```python
from build123d import *

# Parameters (mm, degrees)
ESQUISSE1_R                  = 250
BOSS_EXTRU_1_DEPTH           = 5
D_GAGEMENT_M101_D            = 12
D_GAGEMENT_M101_CSINK_D      = 12.05
D_GAGEMENT_M101_CSINK_ANGLE  = 90
ESQUISSE6_R                  = 1.25
ENL_V_MAT_EXTRU_1_DEPTH      = 11
R_P_TITION_CIRCULAIRE1_COUNT = 3


with BuildPart() as part:
    # Esquisse1 → Boss.-Extru.1 (new body, symmetric)
    with BuildSketch(Plane(origin=(0, 0, 0), x_dir=(1, 0, 0), z_dir=(0, 1, 0))):
        Circle(ESQUISSE1_R)
    extrude(amount=BOSS_EXTRU_1_DEPTH, both=True)

    # Dégagement M101 (through all)
    with Locations(Plane(origin=(0, 5, 0), x_dir=(1, 0, 0), z_dir=(0, 1, 0))):
        with Locations((0, 0)):
            CounterSinkHole(D_GAGEMENT_M101_D / 2, D_GAGEMENT_M101_CSINK_D / 2, counter_sink_angle=D_GAGEMENT_M101_CSINK_ANGLE)

    # Esquisse6 → Enlèv. mat.-Extru.1 (cut, through all)
    with BuildSketch(Plane(origin=(0, 5, 0), x_dir=(1, 0, 0), z_dir=(0, 1, 0))):
        with Locations((200, 8)):
            Circle(ESQUISSE6_R)
        with Locations((200, -8)):
            Circle(ESQUISSE6_R)
    enl_v_mat_extru_1 = extrude(amount=-ENL_V_MAT_EXTRU_1_DEPTH, mode=Mode.SUBTRACT)

    # Répétition circulaire1: Enlèv. mat.-Extru.1 ×3 about axis
    r_p_tition_circulaire1_axis = Axis((0, 0, 0), (0, 1, 0))
    for i in range(1, R_P_TITION_CIRCULAIRE1_COUNT):
        add(enl_v_mat_extru_1.rotate(r_p_tition_circulaire1_axis, i * 360 / R_P_TITION_CIRCULAIRE1_COUNT), mode=Mode.SUBTRACT)


solid = part.part
```
CAD build for the part. Positions are in the model's coordinates, mm. Round coordinates to 2 decimals unless told otherwise and drop trailing zeros. Write each loop counter-clockwise with the first axis right and the second up, starting at its lowest first coordinate (ties: lowest second). Pieces come first, ordered by that corner, then holes. Notation, with made-up numbers: (-34.5, 41) - (-24.5, 41) arc R20 ccw to (-24.5, 78) - close; hole circle Ø7 at (8, 77.25). An arc over 180 degrees is marked (long way). Return JSON: item names as keys, results as strings. Group by question number.
Item 1: Band-saw the part on A-A on z = 0. List the corners of the cut face in (x, y) (3 decimals), plus the area to 3 significant figures.
Item 2: Probe probe 1 along Z at (x, y) = (-93, 1); probe 2 along Z at (x, y) = (0, 1.5); probe 3 along Z at (x, y) = (-5, -0.25). List the from-to ranges inside material, lowest first.
Item 3: Flat gauge pins, fed straight in: pin 1 Ø6 at (y, z) = (1.5, 112.5) entering from +X; pin 2 Ø1.5 at (x, y) = (-129, -2.5) entering from +Z. Where does each tip first touch, or does it go through?
Item 4: Band-saw the part on B-B on x = 0. List the corners of the cut face in (y, z) (3 decimals).
Item 5: Mould opens along Z. For faces 1 (the face through (-249.76, 0.07, -10.99)), 2 (the face through (-3, 5, 52)), 3 (the face through (6, 0, 0)) say: +Z half, -Z half, draft (parallel to the pull), parting line (faces both ways), or undercut.
Item 6: Band-saw the part on D-D on z = 159. List the corners of the cut face in (x, y), plus the area to 3 significant figures.
Item 7: Band-saw the part on C-C on y = -1.5. List the corners of the cut face in (x, z).
Resolved:
{
 "1": {"outline": "(-250, -5) - (-6, -5) - (-6, 4.975) - (-6.025, 5) - (-250, 5) - close; (6, -5) - (250, -5) - (250, 5) - (6.025, 5) - (6, 4.975) - close", "area": "4,880 mm²"},
 "2": {"probe 1": "z = -232.06 to -178.45, -175.96 to 175.96, 178.45 to 232.06", "probe 2": "z = -250 to -6, 6 to 250", "probe 3": "z = -249.95 to -3.32, 3.32 to 249.95"},
 "3": {"pin 1": "stops at x = 224.74", "pin 2": "stops at z = 214.6"},
 "4": {"outline": "(-5, -250) - (5, -250) - (5, -6.025) - (4.975, -6) - (-5, -6) - close; (-5, 6) - (4.975, 6) - (5, 6.025) - (5, 250) - (-5, 250) - close"},
 "5": {"face 1": "parting line", "face 2": "draft", "face 3": "undercut"},
 "6": {"outline": "(-192.92, -5) - (192.92, -5) - (192.92, 5) - (-192.92, 5) - close", "area": "3,860 mm²"},
 "7": {"outline": "circle Ø500 at (0, 0); hole circle Ø2.5 at (-106.93, -169.21); hole circle Ø2.5 at (-106.93, 169.21); hole circle Ø2.5 at (-93.07, -177.21); hole circle Ø2.5 at (-93.07, 177.21); hole circle Ø12 at (0, 0); hole circle Ø2.5 at (200, -8); hole circle Ø2.5 at (200, 8)"}
}
